Can you work these out from the model? Positions are in its coordinate system, mm. Face numbers are marked on the shaded views. A direction names the side the tool comes from. Give positions to 0.01 mm unless a question says otherwise; leave off trailing zeros. Loops run counter-clockwise (first coordinate to the right, second up) from the corner with the lowest first, then second, coordinate; pieces in that order, holes last. Notation, with made-up numbers: (34.5, 62.25) - (47.5, 62.25) arc R17 cw to (47.5, 74.25) - close; hole circle Ø7 at (58, -15.5). An arc over 180 degrees is marked (long way). Answer as a JSON object with one key per item and string values.
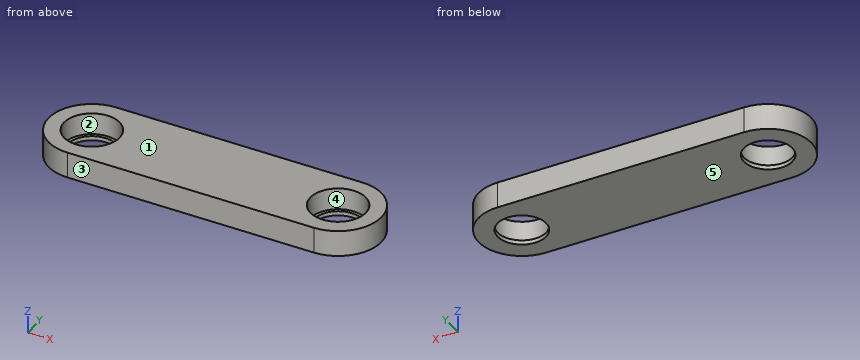
```python
from build123d import *

# Parameters (mm, degrees)
EXTRUDE_1_DEPTH          = 15
SKETCH_2_R               = 16
CUT_EXTRUDE_1_DEPTH      = 12.5
SKETCH_3_R               = 14
CUT_EXTRUDE_2_DEPTH      = 1
CUT_EXTRUDE_2_DEPTH_BACK = 16


with BuildPart() as part:
    # 草图1 → 凸台-拉伸1 (new body)
    with BuildSketch(Plane.XY):
        with BuildLine():
            Line((-72.5, 25), (72.5, 25))
            ThreePointArc((72.5, 25), (97.5, 0), (72.5, -25))
            Line((72.5, -25), (-72.5, -25))
            ThreePointArc((-72.5, -25), (-97.5, 0), (-72.5, 25))
        make_face()
    extrude(amount=EXTRUDE_1_DEPTH)

    # 草图2 → 切除-拉伸1 (cut)
    with BuildSketch(Plane.XY.offset(15)):
        with Locations((-72.5, 0)):
            Circle(SKETCH_2_R)
        with Locations((72.5, 0)):
            Circle(SKETCH_2_R)
    extrude(amount=-CUT_EXTRUDE_1_DEPTH, mode=Mode.SUBTRACT)

    # 草图3 → 切除-拉伸2 (cut, two sides)
    with BuildSketch(Plane.XY.offset(15)) as cut_extrude_2_sk:
        with Locations((-72.5, 0)):
            Circle(SKETCH_3_R)
        with Locations((72.5, 0)):
            Circle(SKETCH_3_R)
    extrude(amount=CUT_EXTRUDE_2_DEPTH, mode=Mode.SUBTRACT)
    extrude(cut_extrude_2_sk.sketch, amount=-CUT_EXTRUDE_2_DEPTH_BACK, mode=Mode.SUBTRACT)


solid = part.part
```
1) Imagine slicing it at D-D on y = -19.5. Write out the boundary of the cut face in (x, z).
Check sheet entries:
{"outline": "(-88.14, 0) - (88.14, 0) - (88.14, 15) - (-88.14, 15) - close"}
2) I need wall thicknesses on L1, parallel to X at y = -7, z = 11.5; L2, parallel to X at y = 12, z = 10.75; L3, parallel to Y at x = 72.5, z = 0.6. Which ranges of each line are inside material? Lowest first, please.
Check sheet entries:
{"L1": "-96.5 to -86.89, -58.11 to 58.11, 86.89 to 96.5", "L2": "-94.43 to -83.08, -61.92 to 61.92, 83.08 to 94.43", "L3": "-25 to -14, 14 to 25"}
3) If we mould it in two halves opening along Y, with no side actions, what happens to the marked faces 3, 4 and 5? For each: released by +Y, released by -Y, zero draft, split by the parting line, or undercut.
Check sheet entries:
{"face 3": "released by -Y", "face 4": "undercut", "face 5": "zero draft"}
4) I'm going to push flat-ended pins straight in: P1, Ø1, axis at x = -47, y = 0.5, coming from the -Z side; P2, Ø19, axis at x = -72.5, y = 0, coming from the +Z side; P3, Ø2, axis at y = -6.5, z = 3, coming from the +X side. Where does each tip first touch, or does it pass through?
Check sheet entries:
{"P1": "z = 0", "P2": "through", "P3": "x = 96.89"}
5) Imagine slicing it at A-A on y = 0. Write out the boundary of the cut face in (x, z).
Check sheet entries:
{"outline": "(-97.5, 0) - (-86.5, 0) - (-86.5, 2.5) - (-88.5, 2.5) - (-88.5, 15) - (-97.5, 15) - close; (-58.5, 0) - (58.5, 0) - (58.5, 2.5) - (56.5, 2.5) - (56.5, 15) - (-56.5, 15) - (-56.5, 2.5) - (-58.5, 2.5) - close; (86.5, 0) - (97.5, 0) - (97.5, 15) - (88.5, 15) - (88.5, 2.5) - (86.5, 2.5) - close"}
6) Imagine slicing it at C-C on z = 10.75. Write out the boundary of the cut face in (x, y).
Check sheet entries:
{"outline": "(-72.5, -25) - (72.5, -25) arc R25 ccw to (72.5, 25) - (-72.5, 25) arc R25 ccw to start; hole circle Ø32 at (-72.5, 0); hole circle Ø32 at (72.5, 0)"}
7) Imagine slicing it at B-B on x = -78. Write out the boundary of the cut face in (y, z), and give its area (3 significant figures).
Check sheet entries:
{"outline": "(-24.39, 0) - (-12.87, 0) - (-12.87, 2.5) - (-15.02, 2.5) - (-15.02, 15) - (-24.39, 15) - close; (12.87, 0) - (24.39, 0) - (24.39, 15) - (15.02, 15) - (15.02, 2.5) - (12.87, 2.5) - close", "area": "292 mm2"}
8) Which directions (+Z, -Z, +X, -X, +Y, -Y) give clear straight access to the entire face, cutting with the end or side of a thin tool? Please do the marked faces 1 and 2.
Check sheet entries:
{"face 1": "+Z, +X, -X, +Y, -Y", "face 2": "+Z"}
